```python
from build123d import *

# Parameters (mm, degrees)
CYLINDER887_R          = 1.25
CYLINDER887_DEPTH      = 7
CYLINDER885_R          = 2.6
CYLINDER885_DEPTH      = 11
CYLINDER885_ROLL_ANGLE = 90
CYLINDER883_R          = 1.25
CYLINDER883_DEPTH      = 4
CYLINDER883_ROLL_ANGLE = 90
CYLINDER884_R          = 5.6
CYLINDER884_DEPTH      = 4
CYLINDER884_ROLL_ANGLE = 90
CYLINDER882_R          = 1.25
CYLINDER882_DEPTH      = 4
CYLINDER882_ROLL_ANGLE = 90
BOX549_W               = 6
BOX549_H               = 4
BOX549_DEPTH           = 22
CYLINDER880_R          = 4
CYLINDER880_DEPTH      = 4
CYLINDER880_ROLL_ANGLE = 90
CYLINDER878_R          = 7
CYLINDER878_DEPTH      = 6
CYLINDER878_ROLL_ANGLE = 90
CYLINDER881_R          = 4
CYLINDER881_DEPTH      = 4
CYLINDER881_ROLL_ANGLE = 90
CYLINDER886_R          = 8
CYLINDER886_DEPTH      = 6
CYLINDER886_ROLL_ANGLE = 90
CHAMFER103_SIZE        = 0.99
CHAMFER104_SIZE        = 0.5


with BuildPart() as cylinder1047:
    # Cylinder887 → Cylinder887 (new body)
    with BuildSketch(Plane(origin=(37, 37.75, -8), x_dir=(1, 0, 0), z_dir=(0, 0, 1))):
        Circle(CYLINDER887_R)
    extrude(amount=CYLINDER887_DEPTH)


with BuildPart() as cylinder1045:
    # Cylinder885 → Cylinder885 (new body)
    with BuildSketch(Plane.XY):
        Circle(CYLINDER885_R)
    extrude(amount=CYLINDER885_DEPTH)


with BuildPart() as cylinder1045_1:
    # Cylinder885 roll: moved
    add(cylinder1045.part.rotate(Axis((0, 0, 0), (1, 0, 0)), CYLINDER885_ROLL_ANGLE))


with BuildPart() as cylinder1045_2:
    # Cylinder885 placement: moved
    add(cylinder1045_1.part.moved(Location((37, 39.75, -11))))


with BuildPart() as cylinder1043:
    # Cylinder883 → Cylinder883 (new body)
    with BuildSketch(Plane.XY):
        Circle(CYLINDER883_R)
    extrude(amount=CYLINDER883_DEPTH)


with BuildPart() as cylinder1043_1:
    # Cylinder883 roll: moved
    add(cylinder1043.part.rotate(Axis((0, 0, 0), (1, 0, 0)), CYLINDER883_ROLL_ANGLE))


with BuildPart() as cylinder1043_2:
    # Cylinder883 placement: moved
    add(cylinder1043_1.part.moved(Location((37, 32.75, -33))))


with BuildPart() as cylinder1044:
    # Cylinder884 → Cylinder884 (new body)
    with BuildSketch(Plane.XY):
        Circle(CYLINDER884_R)
    extrude(amount=CYLINDER884_DEPTH)


with BuildPart() as cylinder1044_1:
    # Cylinder884 roll: moved
    add(cylinder1044.part.rotate(Axis((0, 0, 0), (1, 0, 0)), CYLINDER884_ROLL_ANGLE))


with BuildPart() as cylinder1044_2:
    # Cylinder884 placement: moved
    add(cylinder1044_1.part.moved(Location((37, 39.75, -11))))


with BuildPart() as fusion566:
    # Cylinder882 → Cylinder882 (new body)
    with BuildSketch(Plane.XY):
        Circle(CYLINDER882_R)
    extrude(amount=CYLINDER882_DEPTH)


with BuildPart() as fusion566_1:
    # Cylinder882 roll: moved
    add(fusion566.part.rotate(Axis((0, 0, 0), (1, 0, 0)), CYLINDER882_ROLL_ANGLE))


with BuildPart() as fusion566_2:
    # Cylinder882 placement: moved
    add(fusion566_1.part.moved(Location((37, 32.75, -24))))

    # Fusion566: union Cylinder1045, Cylinder1043, Cylinder1044
    add(cylinder1045_2.part)
    add(cylinder1043_2.part)
    add(cylinder1044_2.part)


with BuildPart() as cube740:
    # Box549 → Box549 (new body)
    with BuildSketch(Plane(origin=(34, 33.75, -33), x_dir=(1, 0, 0), z_dir=(0, 0, 1))):
        with Locations((3, 2)):
            Rectangle(BOX549_W, BOX549_H)
    extrude(amount=BOX549_DEPTH)


with BuildPart() as cylinder1040:
    # Cylinder880 → Cylinder880 (new body)
    with BuildSketch(Plane.XY):
        Circle(CYLINDER880_R)
    extrude(amount=CYLINDER880_DEPTH)


with BuildPart() as cylinder1040_1:
    # Cylinder880 roll: moved
    add(cylinder1040.part.rotate(Axis((0, 0, 0), (1, 0, 0)), CYLINDER880_ROLL_ANGLE))


with BuildPart() as cylinder1040_2:
    # Cylinder880 placement: moved
    add(cylinder1040_1.part.moved(Location((37, 37.75, -33))))


with BuildPart() as cylinder1039:
    # Cylinder878 → Cylinder878 (new body)
    with BuildSketch(Plane.XY):
        Circle(CYLINDER878_R)
    extrude(amount=CYLINDER878_DEPTH)


with BuildPart() as cylinder1039_1:
    # Cylinder878 roll: moved
    add(cylinder1039.part.rotate(Axis((0, 0, 0), (1, 0, 0)), CYLINDER878_ROLL_ANGLE))


with BuildPart() as cylinder1039_2:
    # Cylinder878 placement: moved
    add(cylinder1039_1.part.moved(Location((37, 39.75, -11))))


with BuildPart() as fusion564:
    # Cylinder881 → Cylinder881 (new body)
    with BuildSketch(Plane.XY):
        Circle(CYLINDER881_R)
    extrude(amount=CYLINDER881_DEPTH)


with BuildPart() as fusion564_1:
    # Cylinder881 roll: moved
    add(fusion564.part.rotate(Axis((0, 0, 0), (1, 0, 0)), CYLINDER881_ROLL_ANGLE))


with BuildPart() as fusion564_2:
    # Cylinder881 placement: moved
    add(fusion564_1.part.moved(Location((37, 37.75, -24))))

    # Fusion564: union Cube740, Cylinder1040, Cylinder1039
    add(cube740.part)
    add(cylinder1040_2.part)
    add(cylinder1039_2.part)


with BuildPart() as fusion564_3:
    # Fusion564 placement: moved
    add(fusion564_2.part.moved(Location((0, -5, 0))))


with BuildPart() as front_axle_steering_arm_int_servo:
    # Cylinder886 → Cylinder886 (new body)
    with BuildSketch(Plane.XY):
        Circle(CYLINDER886_R)
    extrude(amount=CYLINDER886_DEPTH)


with BuildPart() as front_axle_steering_arm_int_servo_1:
    # Cylinder886 roll: moved
    add(front_axle_steering_arm_int_servo.part.rotate(Axis((0, 0, 0), (1, 0, 0)), CYLINDER886_ROLL_ANGLE))


with BuildPart() as front_axle_steering_arm_int_servo_2:
    # Cylinder886 placement: moved
    add(front_axle_steering_arm_int_servo_1.part.moved(Location((37, 39.75, -11))))

    # Fusion565: union Fusion564
    add(fusion564_3.part)

    # Cut671: cut Fusion566
    add(fusion566_2.part, mode=Mode.SUBTRACT)

    # Chamfer103
    chamfer103_edges = [front_axle_steering_arm_int_servo_2.edges().sort_by_distance(p)[0] for p in [
        (30, 33.75, -11),
    ]]
    chamfer(chamfer103_edges, length=CHAMFER103_SIZE)

    # Cut672: cut Cylinder1047
    add(cylinder1047.part, mode=Mode.SUBTRACT)

    # Chamfer104
    chamfer104_edges = [front_axle_steering_arm_int_servo_2.edges().sort_by_distance(p)[0] for p in [
        (33.258343, 28.75, -5.08392),
        (42.91608, 28.75, -14.741657),
        (40, 28.75, -19.339402),
        (40.741657, 28.75, -22.585786),
        (34, 28.75, -19.339402),
        (40.741657, 28.75, -25.414214),
        (33, 28.75, -24),
        (40, 28.75, -28.5),
        (34, 28.75, -28.5),
        (40.741657, 28.75, -31.585786),
        (35.585786, 28.75, -36.741657),
        (34, 32.75, -19.339402),
        (40, 32.75, -19.339402),
        (40.741657, 32.75, -22.585786),
        (40.741657, 32.75, -25.414214),
        (40, 32.75, -28.5),
        (33, 32.75, -24),
        (40.741657, 32.75, -31.585786),
        (34, 32.75, -28.5),
        (35.585786, 32.75, -36.741657),
    ]]
    chamfer(chamfer104_edges, length=CHAMFER104_SIZE)


solid = front_axle_steering_arm_int_servo_2.part
```
CAD build for the part. Positions are in the model's coordinates, mm. A direction names the side the tool comes from. Give positions to 0.01 mm unless a question says otherwise; leave off trailing zeros. Write each loop counter-clockwise with the first axis right and the second up, starting at its lowest first coordinate (ties: lowest second). Pieces come first, ordered by that corner, then holes. Notation, with made-up numbers: (59.25, -5) -> (116.25, -5) arc R6 ccw to (116.25, 3) -> close; hole circle Ø9 at (-10.5, 7). An arc over 180 degrees is marked (long way). Write each question's results on one line, items separated by ' | '.
1. Cut at A-A, the plane z = -33. Write the cut outline in (x, y), then the cut area to 3 significant figures.
Geometry check:
outline: (33, 29.25) -> (33.5, 28.75) -> (35.75, 28.75) -> (35.75, 32.75) -> (33.5, 32.75) -> (33, 32.25) -> close; (38.25, 28.75) -> (40.5, 28.75) -> (41, 29.25) -> (41, 32.25) -> (40.5, 32.75) -> (38.25, 32.75) -> close | area: 21.5 mm²
2. Cut at C-C, the plane y = 35.25. Write the cut outline in (x, z), then the cut area to 3 significant figures.
Geometry check:
outline: circle Ø16 at (37, -11); hole circle Ø5.2 at (37, -11) | area: 180 mm²
3. Cut at B-B, the plane x = 37. Give the number of separate pieces and of enclosed holes in the cut face, then the cut area to 3 significant figures.
Geometry check:
separate pieces: 5 | enclosed holes: 0 | area: 135 mm²
4. Cut at D-D, the plane y = 37.75. Write the cut outline in (x, z).
Geometry check:
outline: (35.75, -5.54) -> (35.75, -3.1) arc R8 ccw (long way) to (38.25, -3.1) -> (38.25, -5.54) arc R5.6 cw (long way) to start
5. Two-plate mould, pull along Y, no slides. Class faces 1 (the conical face through (37.12, 28.89, -36.64)), 2 (the cylindrical face through (37, 31, -37)), 3 (the cylindrical face through (38.2, 38.1, -4.3)): pulls with the +Y half, pulls with the -Y half, needs draft (parallel to the pull), parting line crosses it, or undercut.
Geometry check:
face 1: pulls with the -Y half | face 2: needs draft | face 3: undercut
6. Wall check: probe 1 along Z at (x, y) = (37, 31); probe 2 along X at (y, z) = (32.5, -11); probe 3 along X at (y, z) = (30.3, -33). Give the ranges that are in metal, low to high. Write a range as [from, to].
Geometry check:
probe 1: [-37, -34.25], [-31.75, -25.25], [-22.75, -13.6], [-8.4, -4] | probe 2: [30, 34.4], [39.6, 44] | probe 3: [33, 35.75], [38.25, 41]
7. Drop flat-ended pins along their axis: P1, Ø3, axis at x = 37, y = 37.75, coming from the +Z side; P2, Ø3, axis at y = 31, z = -32, coming from the -X side; P3, Ø1.5, axis at x = 38, z = -13.5, coming from the +Y side; P4, Ø1.5, axis at x = 37, z = -33, coming from the -Y side. Give the stop position or say it passes through.
Geometry check:
P1: z = -3 | P2: x = 33 | P3: y = 35.75 | P4: through
8. Which spindle directions (+Z, -Z, +X, -X, +Y, -Y) get a long thin tool onto all of the face, cutting with end or side? Do faces 4 (the flat face through (40, 31, -29)), 5 (the flat face through (40, 31, -19)), 6 (the flat face through (34, 31, -29)). Say none if no direction does.
Geometry check:
face 4: +X, +Y, -Y | face 5: +X, -Y | face 6: -X, +Y, -Y
